```python
from build123d import *

# Parameters (mm, degrees)
CUT_EXTRUDE_1_DEPTH = 2.5
CUT_EXTRUDE_2_DEPTH = 3
CUT_EXTRUDE_4_DEPTH = 29.722813233
SKETCH_8_R          = 2.05
CUT_EXTRUDE_6_DEPTH = 5


with BuildPart() as part:
    # 草图2 → 旋转1 (revolve)
    with BuildSketch(Plane.XY, mode=Mode.PRIVATE) as revolve_1_sk:
        with BuildLine():
            Line((3, 8), (3, 0))
            Line((3, 0), (20, 0))
            Line((20, 0), (20, 1.210446983))
            ThreePointArc((20, 1.210446983), (18.95, 3), (20, 4.789553017))
            Line((20, 4.789553017), (20, 8))
            Line((20, 8), (3, 8))
        make_face()
    revolve(revolve_1_sk.sketch.rotate(Axis((0, 0, 0), (0, 1, 0)), 90), axis=Axis((0, 0, 0), (0, 1, 0)))

    # 草图3 → 切除-拉伸1 (cut)
    with BuildSketch(Plane.XZ):
        with BuildLine():
            Line((1.835992055, -17.350058041), (3.408354199, -10.798521635))
            ThreePointArc((3.408354199, -10.798521635), (6.061153739, -6.061181984), (10.798487471, -3.408371874))
            Line((10.798487471, -3.408371874), (17.350061912, -1.835985141))
            ThreePointArc((17.350061912, -1.835985141), (18.129967792, -1.363900547), (18.492480347, -0.527418811))
            Line((18.492480347, -0.527418811), (18.492480347, 0.527418811))
            ThreePointArc((18.492480347, 0.527418811), (18.129968102, 1.363905618), (17.350058041, 1.835992055))
            Line((17.350058041, 1.835992055), (10.798521635, 3.408354199))
            ThreePointArc((10.798521635, 3.408354199), (6.061181984, 6.061153739), (3.408371874, 10.798487471))
            Line((3.408371874, 10.798487471), (1.835985141, 17.350061912))
            ThreePointArc((1.835985141, 17.350061912), (1.363900547, 18.129967792), (0.527418811, 18.492480347))
            Line((0.527418811, 18.492480347), (-0.527418811, 18.492480347))
            ThreePointArc((-0.527418811, 18.492480347), (-1.363905618, 18.129968102), (-1.835992055, 17.350058041))
            Line((-1.835992055, 17.350058041), (-3.408354199, 10.798521635))
            ThreePointArc((-3.408354199, 10.798521635), (-6.061153739, 6.061181984), (-10.798487471, 3.408371874))
            Line((-10.798487471, 3.408371874), (-17.350061912, 1.835985141))
            ThreePointArc((-17.350061912, 1.835985141), (-18.129967792, 1.363900547), (-18.492480347, 0.527418811))
            Line((-18.492480347, 0.527418811), (-18.492480347, -0.527418811))
            ThreePointArc((-18.492480347, -0.527418811), (-18.129968102, -1.363905618), (-17.350058041, -1.835992055))
            Line((-17.350058041, -1.835992055), (-10.798521635, -3.408354199))
            ThreePointArc((-10.798521635, -3.408354199), (-6.061181984, -6.061153739), (-3.408371874, -10.798487471))
            Line((-3.408371874, -10.798487471), (-1.835985141, -17.350061912))
            ThreePointArc((-1.835985141, -17.350061912), (-1.363900547, -18.129967792), (-0.527418811, -18.492480347))
            Line((-0.527418811, -18.492480347), (0.527418811, -18.492480347))
            ThreePointArc((0.527418811, -18.492480347), (1.363905618, -18.129968102), (1.835992055, -17.350058041))
        make_face()
    extrude(amount=-CUT_EXTRUDE_1_DEPTH, mode=Mode.SUBTRACT)

    # 草图4 → 切除-拉伸2 (cut)
    with BuildSketch(Plane.XZ):
        Polygon((13.485234102, 9.96339746), (11.810918321, 12.86339746), (8.46228676, 12.86339746), (6.787970979, 9.96339746), (8.46228676, 7.06339746), (11.810918321, 7.06339746), align=None)
        Polygon((-10, 13.348631561), (-12.9, 11.674315781), (-12.9, 8.325684219), (-10, 6.651368439), (-7.1, 8.325684219), (-7.1, 11.674315781), align=None)
        Polygon((10.1, -13.521836642), (13, -11.847520861), (13, -8.4988893), (10.1, -6.824573519), (7.2, -8.4988893), (7.2, -11.847520861), align=None)
        Polygon((-13.385234102, -10.13660254), (-11.710918321, -13.03660254), (-8.36228676, -13.03660254), (-6.687970979, -10.13660254), (-8.36228676, -7.23660254), (-11.710918321, -7.23660254), align=None)
    extrude(amount=-CUT_EXTRUDE_2_DEPTH, mode=Mode.SUBTRACT)

    # 草图6 → 切除-拉伸4 (cut, through all)
    with BuildSketch(Plane.XZ.offset(-3)):
        with BuildLine():
            Line((-10, -8), (-10, -10))
            Line((-10, -10), (-8, -10))
            ThreePointArc((-8, -10), (-8.585786438, -8.585786438), (-10, -8))
        make_face()
        with BuildLine():
            Line((-8, -10), (-10, -10))
            Line((-10, -10), (-10, -8))
            ThreePointArc((-10, -8), (-11.414213562, -11.414213562), (-8, -10))
        make_face()
        with BuildLine():
            ThreePointArc((-8, 10), (-11.414213562, 11.414213562), (-10, 8))
            Line((-10, 8), (-10, 10))
            Line((-10, 10), (-8, 10))
        make_face()
        with BuildLine():
            Line((-10, 10), (-10, 8))
            ThreePointArc((-10, 8), (-8.585786438, 8.585786438), (-8, 10))
            Line((-8, 10), (-10, 10))
        make_face()
        with BuildLine():
            ThreePointArc((8, 10), (8.585786438, 8.585786438), (10, 8))
            Line((10, 8), (10, 10))
            Line((10, 10), (8, 10))
        make_face()
        with BuildLine():
            Line((10, 10), (10, 8))
            ThreePointArc((10, 8), (11.414213562, 8.585786438), (12, 10))
            ThreePointArc((12, 10), (10, 12), (8, 10))
            Line((8, 10), (10, 10))
        make_face()
        with BuildLine():
            ThreePointArc((10, -8), (8.585786438, -8.585786438), (8, -10))
            Line((8, -10), (10, -10))
            Line((10, -10), (10, -8))
        make_face()
        with BuildLine():
            Line((10, -10), (8, -10))
            ThreePointArc((8, -10), (10, -12), (12, -10))
            ThreePointArc((12, -10), (11.414213562, -8.585786438), (10, -8))
            Line((10, -8), (10, -10))
        make_face()
    extrude(amount=-CUT_EXTRUDE_4_DEPTH, mode=Mode.SUBTRACT)

    # 草图8 → 切除-拉伸6 (cut)
    with BuildSketch(Plane(origin=(0, 8, 0), x_dir=(1, 0, 0), z_dir=(0, 1, 0))):
        with Locations((0, 21)):
            Circle(SKETCH_8_R)
    extrude(amount=-CUT_EXTRUDE_6_DEPTH, mode=Mode.SUBTRACT)


solid = part.part
```
Work out the finished part from the listing and answer in its coordinate system (mm). A direction names the side the tool comes from. Round coordinates to 2 decimals unless told otherwise and drop trailing zeros. Write each loop counter-clockwise with the first axis right and the second up, starting at its lowest first coordinate (ties: lowest second). Pieces come first, ordered by that corner, then holes.
1) A cutting plane is placed at C-C on x = -9.5. Give the number of separate pieces and of enclosed holes in the cut face, and give its area (3 significant figures).
2) A cutting plane is placed at A-A on x = 0. Determine the outline of the cut face in (y, z), and give its area (3 significant figures).
3) A cutting plane is placed at B-B on y = 7.5. Determine the outline of the cut face in (x, z).
4) Which of the six approach directions +Z, -Z, +X, -X, +Y, -Y give full straight-line access (tool end or side, diameter ignored) to faces 1 (the face through (-0.9, 5.21, -2.86)), 2 (the face through (18.1, 1.2, -1.4)), 3 (the face through (-0.03, 6.09, -18.95))?
5) Consider probe 1 along X at (y, z) = (2.25, 7); probe 2 along Z at (x, y) = (-10, 5.15); probe 3 along X at (y, z) = (2, 9). Determine where each line is inside the solid, lowest interval first.
6) Flat-ended cylindrical pins translate along their axes: P1, Ø2.5, axis at y = 1.5, z = 10, coming from the -X side; P2, Ø5.5, axis at x = 0, z = 0, coming from the +Y side; P3, Ø2, axis at y = 4, z = -13, coming from the -X side; P4, Ø8, axis at x = -6.5, z = 13.5, coming from the -Y side. Find the tip coordinate at first contact, or state that the pin passes through.
7) Determine the mould class of faces 4 (the face through (7.637, 1.479, 11.434)), 5 (the face through (0, 8, -4)) for opening direction X: pulls with the +X half, pulls with the -X half, needs draft (parallel to the pull), parting line crosses it, or undercut.
Entries:
1. separate pieces: 3
1. enclosed holes: 0
1. area: 182 mm2
2. outline: (0, -20) - (1.21, -20) arc R2.05 cw to (3, -18.95) - (8, -18.95) - (8, -3) - (2.5, -3) - (2.5, -18.49) - (0, -18.49) - close; (0, 18.49) - (2.5, 18.49) - (2.5, 3) - (8, 3) - (8, 20) - (4.79, 20) arc R2.05 cw to (1.21, 20) - (0, 20) - close
2. area: 185 mm2
3. outline: (-1.74, -19.92) arc R2.05 cw to (1.74, -19.92) arc R20 ccw (long way) to start; hole circle Ø4 at (-10, -10); hole circle Ø4 at (-10, 10); hole circle Ø6 at (0, 0); hole circle Ø4 at (10, -10); hole circle Ø4 at (10, 10)
4. face 1: +Y, -Y
4. face 2: -Y
4. face 3: -Z, +Y
5. probe 1: x = -17.76 to -10.6, -9.4 to -5.23, 5.23 to 17.76
5. probe 2: z = -17.32 to -12, -8 to 8, 12 to 17.32
5. probe 3: x = -16.97 to -12.9, -7.1 to -4.03, 4.03 to 7.34, 12.93 to 16.97
6. P1: stops at x = -17.97
6. P2: passes through
6. P3: stops at x = -15.7
6. P4: stops at y = 0
7. face 4: undercut
7. face 5: needs draft
